For this review, take the finished solid that the model builds, in its own axes (mm). Round coordinates to 2 decimals unless told otherwise and drop trailing zeros. Order: outer loops, then holes, each group sorted by start corner. A loop starts at its lowest first (then second) coordinate and runs counter-clockwise, first axis right, second up.
```python
from build123d import *

# Parameters (mm, degrees)
SKETCH2_R           = 7.9375
SKETCH2_R_2         = 3.81
SKETCH2_R_3         = 3.302
SKETCH2_W           = 12.446
SKETCH2_H           = 6.35
SKETCH2_W_2         = 6.35
SKETCH2_H_2         = 12.446
BOSS_EXTRUDE1_DEPTH = 6.35


with BuildPart() as part:
    # Sketch2 → Boss-Extrude1 (new body)
    with BuildSketch(Plane(origin=(0, 0, 0), x_dir=(1, 0, 0), z_dir=(0, 1, 0))):
        with BuildLine():
            Line((-114.3, -165.1), (114.3, -165.1))
            ThreePointArc((114.3, -165.1), (150.221024484, -150.221024484), (165.1, -114.3))
            Line((165.1, -114.3), (165.1, 114.3))
            ThreePointArc((165.1, 114.3), (150.221024484, 150.221024484), (114.3, 165.1))
            Line((114.3, 165.1), (-114.3, 165.1))
            ThreePointArc((-114.3, 165.1), (-150.221024484, 150.221024484), (-165.1, 114.3))
            Line((-165.1, 114.3), (-165.1, -114.3))
            ThreePointArc((-165.1, -114.3), (-150.221024484, -150.221024484), (-114.3, -165.1))
        make_face()
        Circle(SKETCH2_R, mode=Mode.SUBTRACT)
        with Locations((25.4, -25.4)):
            Circle(SKETCH2_R_2, mode=Mode.SUBTRACT)
        with Locations((25.4, 25.4)):
            Circle(SKETCH2_R_2, mode=Mode.SUBTRACT)
        with Locations((-25.4, 25.4)):
            Circle(SKETCH2_R_2, mode=Mode.SUBTRACT)
        with Locations((-25.4, -25.4)):
            Circle(SKETCH2_R_2, mode=Mode.SUBTRACT)
        with Locations((133.35, -28.575)):
            Circle(SKETCH2_R_3, mode=Mode.SUBTRACT)
        with Locations((-133.35, -28.575)):
            Circle(SKETCH2_R_3, mode=Mode.SUBTRACT)
        with Locations((-133.35, 28.575)):
            Circle(SKETCH2_R_3, mode=Mode.SUBTRACT)
        with Locations((133.35, 28.575)):
            Circle(SKETCH2_R_3, mode=Mode.SUBTRACT)
        with BuildLine():
            Line((-123.19, 128.27), (-36.83, 128.27))
            ThreePointArc((-36.83, 128.27), (-33.237897552, 126.782102448), (-31.75, 123.19))
            Line((-31.75, 123.19), (-31.75, 36.83))
            ThreePointArc((-31.75, 36.83), (-33.237897552, 33.237897552), (-36.83, 31.75))
            Line((-36.83, 31.75), (-123.19, 31.75))
            ThreePointArc((-123.19, 31.75), (-126.782102448, 33.237897552), (-128.27, 36.83))
            Line((-128.27, 36.83), (-128.27, 123.19))
            ThreePointArc((-128.27, 123.19), (-126.782102448, 126.782102448), (-123.19, 128.27))
        make_face(mode=Mode.SUBTRACT)
        with BuildLine():
            Line((36.83, 128.27), (123.19, 128.27))
            ThreePointArc((123.19, 128.27), (126.782102448, 126.782102448), (128.27, 123.19))
            Line((128.27, 123.19), (128.27, 36.83))
            ThreePointArc((128.27, 36.83), (126.782102448, 33.237897552), (123.19, 31.75))
            Line((123.19, 31.75), (36.83, 31.75))
            ThreePointArc((36.83, 31.75), (33.237897552, 33.237897552), (31.75, 36.83))
            Line((31.75, 36.83), (31.75, 123.19))
            ThreePointArc((31.75, 123.19), (33.237897552, 126.782102448), (36.83, 128.27))
        make_face(mode=Mode.SUBTRACT)
        with BuildLine():
            Line((-123.19, -31.75), (-36.83, -31.75))
            ThreePointArc((-36.83, -31.75), (-33.237897552, -33.237897552), (-31.75, -36.83))
            Line((-31.75, -36.83), (-31.75, -123.19))
            ThreePointArc((-31.75, -123.19), (-33.237897552, -126.782102448), (-36.83, -128.27))
            Line((-36.83, -128.27), (-123.19, -128.27))
            ThreePointArc((-123.19, -128.27), (-126.782102448, -126.782102448), (-128.27, -123.19))
            Line((-128.27, -123.19), (-128.27, -36.83))
            ThreePointArc((-128.27, -36.83), (-126.782102448, -33.237897552), (-123.19, -31.75))
        make_face(mode=Mode.SUBTRACT)
        with BuildLine():
            Line((36.83, -31.75), (123.19, -31.75))
            ThreePointArc((123.19, -31.75), (126.782102448, -33.237897552), (128.27, -36.83))
            Line((128.27, -36.83), (128.27, -123.19))
            ThreePointArc((128.27, -123.19), (126.782102448, -126.782102448), (123.19, -128.27))
            Line((123.19, -128.27), (36.83, -128.27))
            ThreePointArc((36.83, -128.27), (33.237897552, -126.782102448), (31.75, -123.19))
            Line((31.75, -123.19), (31.75, -36.83))
            ThreePointArc((31.75, -36.83), (33.237897552, -33.237897552), (36.83, -31.75))
        make_face(mode=Mode.SUBTRACT)
        with Locations((-127, -142.875)):
            Rectangle(SKETCH2_W, SKETCH2_H, mode=Mode.SUBTRACT)
        with Locations((127, -142.875)):
            Rectangle(SKETCH2_W, SKETCH2_H, mode=Mode.SUBTRACT)
        with Locations((-142.875, 127)):
            Rectangle(SKETCH2_W_2, SKETCH2_H_2, mode=Mode.SUBTRACT)
        with Locations((-142.875, -127)):
            Rectangle(SKETCH2_W_2, SKETCH2_H_2, mode=Mode.SUBTRACT)
        with Locations((127, 142.875)):
            Rectangle(SKETCH2_W, SKETCH2_H, mode=Mode.SUBTRACT)
        with Locations((-127, 142.875)):
            Rectangle(SKETCH2_W, SKETCH2_H, mode=Mode.SUBTRACT)
        with Locations((142.875, -127)):
            Rectangle(SKETCH2_W_2, SKETCH2_H_2, mode=Mode.SUBTRACT)
        with Locations((142.875, 127)):
            Rectangle(SKETCH2_W_2, SKETCH2_H_2, mode=Mode.SUBTRACT)
    extrude(amount=BOSS_EXTRUDE1_DEPTH)


solid = part.part
```
Q1. Take a section at C-C, the plane y = 3.75. Count the separate pieces of the cut face and the enclosed holes in it, plus the area to 3 significant figures.
Q2. Clearance check with flat-ended pins moving along their axes: pin 1 (3 mm diameter, centred on x = -142.5, y = 4, fed in from +Z); pin 2 (4 mm diameter, centred on x = -49.5, z = 19, fed in from -Y); pin 3 (3 mm diameter, centred on y = 4.5, z = 126, fed in from +X); pin 4 (1.9 mm diameter, centred on y = 4, z = -144, fed in from +X). State where each tip first meets the part, or that it passes through.
Q3. Take a section at B-B, the plane z = 0. State the section outline as (x, y) points, plus the area to 3 significant figures.
Q4. Mouldability with a two-part tool opening along X and no side actions: class faces 1 (the face through (-1.72, 3.13, 7.75)), 2 (the face through (-28.42, 3.13, 27.72)), 3 (the face through (-149.824, 3.131, -150.614)), 4 (the face through (-2, 0, -39)) as +X half, -X half, draft (parallel to the pull), parting line (faces both ways), or undercut.
Q5. Wall thickness on line 1 (Z direction, x = -90, y = 1.75); line 2 (Z direction, x = -25.4, y = 3.25): over which ranges is each line inside the solid? List them lowest first.
Q6. Take a section at A-A, the plane x = 25.4. State the section outline as (y, z) points.
Working result:
1. separate pieces: 1
1. enclosed holes: 21
1. area: 68,500 mm2
2. pin 1: stops at z = 157.52
2. pin 2: stops at y = 0
2. pin 3: stops at x = 164.07
2. pin 4: stops at x = 156.18
3. outline: (-165.1, 0) - (-7.94, 0) - (-7.94, 6.35) - (-165.1, 6.35) - close; (7.94, 0) - (165.1, 0) - (165.1, 6.35) - (7.94, 6.35) - close
3. area: 2,000 mm2
4. face 1: undercut
4. face 2: undercut
4. face 3: -X half
4. face 4: draft
5. line 1: z = -165.1 to -128.27, -31.75 to 31.75, 128.27 to 165.1
5. line 2: z = -165.1 to -29.21, -21.59 to 21.59, 29.21 to 165.1
6. outline: (0, -165.1) - (6.35, -165.1) - (6.35, -29.21) - (0, -29.21) - close; (0, -21.59) - (6.35, -21.59) - (6.35, 21.59) - (0, 21.59) - close; (0, 29.21) - (6.35, 29.21) - (6.35, 165.1) - (0, 165.1) - close
